```python
from build123d import *

# Parameters (mm, degrees)
F0_W     = 550
F0_H     = 550
F1_DEPTH = 15
F2_R     = 200
F3_DEPTH = 5
F4_W     = 50
F4_H     = 50
F5_DEPTH = 15


with BuildPart() as f1:
    # F0 (on Top) → F1 (new body)
    with BuildSketch(Plane.XY):
        Rectangle(F0_W, F0_H)
    extrude(amount=F1_DEPTH)

    # F2 (on face) → F3 (cut)
    with BuildSketch(Plane.XY.offset(15)):
        Circle(F2_R)
    extrude(amount=-F3_DEPTH, mode=Mode.SUBTRACT)

    # F4 (on face) → F5 (cut, through all)
    with BuildSketch(Plane(origin=(0, 0, 0), x_dir=(1, 0, 0), z_dir=(0, 0, -1))):
        with Locations((-250, 250)):
            Rectangle(F4_W, F4_H)
        with Locations((250, 250)):
            Rectangle(F4_W, F4_H)
        with Locations((-250, -250)):
            Rectangle(F4_W, F4_H)
        with Locations((250, -250)):
            Rectangle(F4_W, F4_H)
    extrude(amount=-F5_DEPTH, mode=Mode.SUBTRACT)


solid = f1.part
```
For this review, take the finished solid that the model builds, in its own axes (mm). A direction names the side the tool comes from. Coordinates: 2 decimals unless noted, no trailing zeros. Order: outer loops, then holes, each group sorted by start corner. A loop starts at its lowest first (then second) coordinate and runs counter-clockwise, first axis right, second up. Notation, with made-up numbers: (-4.75, 10) - (28.25, 10) arc R20 ccw to (28.25, 31) - close; hole circle Ø1 at (79, -35.5). An arc over 180 degrees is marked (long way). Answer as a JSON object with one key per item and string values. Group by question number.
1. We need section C-C on z = 5. State the section outline as (x, y) points.
2. We need section A-A on y = 0. State the section outline as (x, z) points, then the cut area to 3 significant figures.
3. We need section D-D on x = -239. State the section outline as (y, z) points, then the cut area to 3 significant figures.
4. Clearance check with flat-ended pins moving along their axes: P1, Ø7.5, axis at y = 245.5, z = 6, coming from the +X side; P2, Ø7.5, axis at y = -250, z = 7.5, coming from the -X side. State where each tip first meets the part, or that it passes through.
5. For faces 1 (the flat face through (-225, -250, 7)), 2 (the flat face through (250, 225, 7)), 3 (the flat face through (-250, 225, 7)), 4 (the flat face through (275, -3, 7)), 5 (the flat face through (250, -225, 7)), list the 3-axis set-ups (+Z, -Z, +X, -X, +Y, -Y) from which the entire face can be reached by the end or side of a thin tool; tool diameter is ignored.
6. For probe 1 along Y at (x, z) = (0, 11.45); probe 2 along Z at (x, y) = (-82, -75.5); probe 3 along X at (y, z) = (-104.5, 11.5), list the stretches that pass through material, from the lowest coordinate up.
7. The part is to be moulded in two halves that separate along X. For faces 6 (the flat face through (-3, 275, 7)), 7 (the cylindrical face through (190.764, 60.075, 12.535)), 8 (the flat face through (-3, 3, 10)), 9 (the flat face through (-225, 250, 7)), say which applies: pulls with the +X half, pulls with the -X half, needs draft (parallel to the pull), parting line crosses it, or undercut.
Final values:
{
 "1": {"outline": "(-275, -225) - (-225, -225) - (-225, -275) - (225, -275) - (225, -225) - (275, -225) - (275, 225) - (225, 225) - (225, 275) - (-225, 275) - (-225, 225) - (-275, 225) - close"},
 "2": {"outline": "(-275, 0) - (275, 0) - (275, 15) - (200, 15) - (200, 10) - (-200, 10) - (-200, 15) - (-275, 15) - close", "area": "6,250 mm²"},
 "3": {"outline": "(-225, 0) - (225, 0) - (225, 15) - (-225, 15) - close", "area": "6,750 mm²"},
 "4": {"P1": "x = 225", "P2": "x = -225"},
 "5": {"face 1": "+Z, -Z, -X, -Y", "face 2": "+Z, -Z, +X, +Y", "face 3": "+Z, -Z, -X, +Y", "face 4": "+Z, -Z, +X, +Y, -Y", "face 5": "+Z, -Z, +X, -Y"},
 "6": {"probe 1": "-275 to -200, 200 to 275", "probe 2": "0 to 10", "probe 3": "-275 to -170.53, 170.53 to 275"},
 "7": {"face 6": "needs draft", "face 7": "undercut", "face 8": "undercut", "face 9": "pulls with the -X half"}
}
